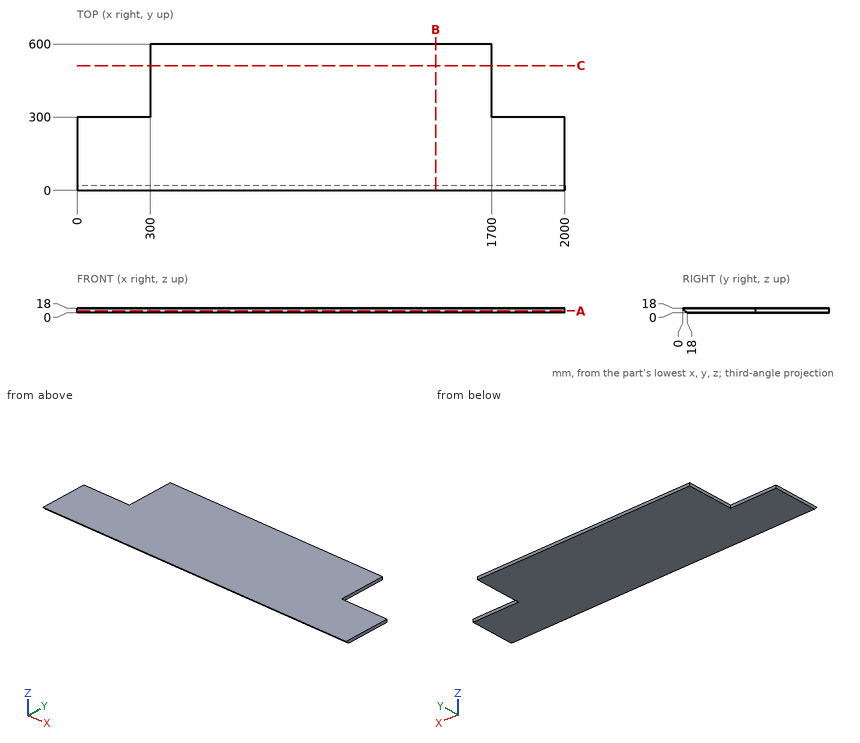
Check sheet for the drawn part. Datum: minimum x, y, z corner. Units: mm. Coordinates: 2 decimals unless noted, no trailing zeros. Loops run counter-clockwise (first coordinate to the right, second up) from the corner with the lowest first, then second, coordinate; pieces in that order, holes last. Notation, with made-up numbers: M -35.5,16 L -14.5,16 A11 ccw -14.5,30 Z; hole C 74.5,37 d4. An arc over 180 degrees is marked long. Answer as a JSON object with one key per item and string values.
1. Depth check by flat-ended pin: P1, Ø3, axis at y = 392, z = 14, coming from the -X side; P2, Ø10, axis at x = 948, z = 3.5, coming from the -Y side; P3, Ø4, axis at x = 880.5, z = 15.5, coming from the -Y side. Enter the tip coordinate at first touch or a pass-through.
Outcome:
{"P1": "x = 300", "P2": "y = 9.5", "P3": "y = 0.5"}
2. Scan lines: L1, parallel to X at y = 484, z = 14; L2, parallel to Y at x = 1546, z = 3.75; L3, parallel to Y at x = 440.5, z = 15.75. Record each from-to range of solid material in increasing order. Write a range as from..to.
Outcome:
{"L1": "300..1700", "L2": "14.25..600", "L3": "2.25..600"}
3. Sectioned sample at C-C on y = 511.5. Record the cut outline in (x, z).
Outcome:
{"outline": "M 300,0 L 1700,0 L 1700,18 L 300,18 Z"}
4. Sectioned sample at A-A on z = 7.75. Record the cut outline in (x, y), and give its area (4 significant figures).
Outcome:
{"outline": "M 0,10.25 L 2000,10.25 L 2000,300 L 1700,300 L 1700,600 L 300,600 L 300,300 L 0,300 Z", "area": "999,500 mm²"}
5. Sectioned sample at B-B on x = 1471. Record the cut outline in (y, z), and give its area (3 significant figures).
Outcome:
{"outline": "M 0,18 L 18,0 L 600,0 L 600,18 Z", "area": "10,600 mm²"}
